Print and shaded views of the part. All mm, measured from the part's lowest x, y and z. A direction names the side the tool comes from. Give positions to 0.01 mm unless a question says otherwise; leave off trailing zeros. Loops run counter-clockwise (first coordinate to the right, second up) from the corner with the lowest first, then second, coordinate; pieces in that order, holes last. Notation, with made-up numbers: M 62,68 L 90,68 A30 cw 90,100 Z; hole C 13.5,26.25 d2. An arc over 180 degrees is marked long. Answer as CSV lines item,"result".
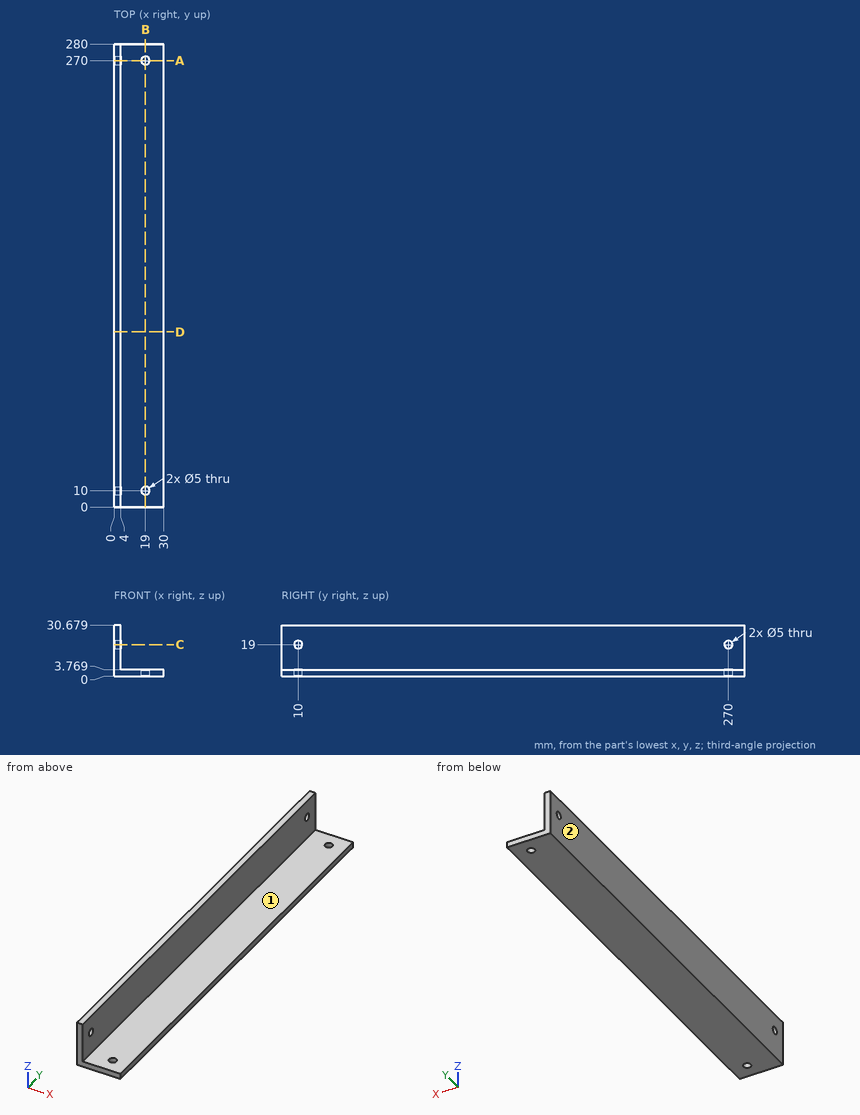
Q1. Cut at C-C (z = 19). Write the cut outline in (x, y), and give its area (3 significant figures).
Solution:
outline,"M 0,0 L 4,0 L 4,7.5 L 0,7.5 Z; M 0,12.5 L 4,12.5 L 4,267.5 L 0,267.5 Z; M 0,272.5 L 4,272.5 L 4,280 L 0,280 Z"
area,"1,080 mm²"
Q2. Cut at D-D (y = 106). Write the cut outline in (x, z), and give its area (3 significant figures).
Solution:
outline,"M 0,0 L 30,0 L 30,3.77 L 4,3.77 L 4,30.68 L 0,30.68 Z"
area,"221 mm²"
Q3. Cut at A-A (y = 270). Write the cut outline in (x, z).
Solution:
outline,"M 0,0 L 16.5,0 L 16.5,3.77 L 4,3.77 L 4,16.5 L 0,16.5 Z; M 0,21.5 L 4,21.5 L 4,30.68 L 0,30.68 Z; M 21.5,0 L 30,0 L 30,3.77 L 21.5,3.77 Z"
Q4. Cut at B-B (x = 19). Write the cut outline in (y, z), and give its area (3 significant figures).
Solution:
outline,"M 0,0 L 7.5,0 L 7.5,3.77 L 0,3.77 Z; M 12.5,0 L 267.5,0 L 267.5,3.77 L 12.5,3.77 Z; M 272.5,0 L 280,0 L 280,3.77 L 272.5,3.77 Z"
area,"1,020 mm²"
Q5. Which spindle directions (+Z, -Z, +X, -X, +Y, -Y) get a long thin tool onto all of the face, cutting with end or side? Do the marked faces 1 and 2. Say none if no direction does.
Solution:
face 1,"+Z, +X, +Y, -Y"
face 2,"+Z, -Z, -X, +Y, -Y"
Q6. Wall check: line 1 (Y direction, x = 1.7, z = 19); line 2 (X direction, y = 270, z = 3); line 3 (Z direction, x = 1.1, y = 270). Give the ranges that are in metal, low to high. Write a range as [from, to].
Solution:
line 1,"y = [0, 7.5], [12.5, 267.5], [272.5, 280]"
line 2,"x = [0, 16.5], [21.5, 30]"
line 3,"z = [0, 16.5], [21.5, 30.68]"
Q7. Pin check, flat tips, straight feed: P1, Ø1, axis at x = 20.5, y = 208.5, coming from the +Z side; P2, Ø8, axis at y = 10, z = 19, coming from the +X side. Stop position of each tip, or through.
Solution:
P1,"stops at z = 3.77"
P2,"stops at x = 4"
